```python
from build123d import *

# Parameters (mm, degrees)
SKETCH_1_R         = 7.5
EXTRUDE_1_DEPTH    = 4.5
SKETCH_9_R         = 2.25
EXTRUDE_6_DEPTH    = 1
EXTRUDE_2_DEPTH    = 5
SKETCH_6_R         = 1.75
EXTRUDE_3_DEPTH    = 0.5
SKETCH_7_R         = 1.5
EXTRUDE_4_DEPTH    = 5
SKETCH_8_R         = 8.5
SKETCH_8_R_2       = 7.5
EXTRUDE_5_DEPTH    = 1
HOLE_WIZARD_M3_1_D = 3.4


with BuildPart() as part:
    # ｽｹｯﾁ1 → ﾎﾞｽ - 押し出し1 (new body)
    with BuildSketch(Plane(origin=(0, 0, 0), x_dir=(1, 0, 0), z_dir=(0, 1, 0))):
        Circle(SKETCH_1_R)
    extrude(amount=EXTRUDE_1_DEPTH)

    # ｽｹｯﾁ9 → ﾎﾞｽ - 押し出し6 (add)
    with BuildSketch(Plane(origin=(0, 4.5, 0), x_dir=(1, 0, 0), z_dir=(0, 1, 0))):
        Circle(SKETCH_9_R)
    extrude(amount=EXTRUDE_6_DEPTH)

    # ｽｹｯﾁ2 → ﾎﾞｽ - 押し出し2 (add)
    with BuildSketch(Plane(origin=(0, 5.5, 0), x_dir=(1, 0, 0), z_dir=(0, 1, 0))):
        Polygon((2.020725942, 0), (1.010362971, 1.75), (-1.010362971, 1.75), (-2.020725942, 0), (-1.010362971, -1.75), (1.010362971, -1.75), align=None)
    extrude(amount=EXTRUDE_2_DEPTH)

    # ｽｹｯﾁ6 → ﾎﾞｽ - 押し出し3 (add)
    with BuildSketch(Plane(origin=(0, 10.5, 0), x_dir=(1, 0, 0), z_dir=(0, 1, 0))):
        Circle(SKETCH_6_R)
    extrude(amount=EXTRUDE_3_DEPTH)

    # ｽｹｯﾁ7 → ﾎﾞｽ - 押し出し4 (add)
    with BuildSketch(Plane(origin=(0, 11, 0), x_dir=(1, 0, 0), z_dir=(0, 1, 0))):
        Circle(SKETCH_7_R)
    extrude(amount=EXTRUDE_4_DEPTH)

    # ｽｹｯﾁ8 → ﾎﾞｽ - 押し出し5 (add)
    with BuildSketch(Plane(origin=(0, 0, 0), x_dir=(-1, 0, 0), z_dir=(0, -1, 0))):
        Circle(SKETCH_8_R)
        Circle(SKETCH_8_R_2, mode=Mode.SUBTRACT)
    extrude(amount=-EXTRUDE_5_DEPTH)

    # M3 すきま穴1 (through all)
    with Locations(Plane(origin=(0, 4.5, 0), x_dir=(1, 0, 0), z_dir=(0, 1, 0))):
        with Locations((0, 6), (0, -6)):
            Hole(HOLE_WIZARD_M3_1_D / 2)


solid = part.part
```
Verification items for the finished model (mm, model axes). A direction names the side the tool comes from. Give positions to 0.01 mm unless a question says otherwise; leave off trailing zeros. Write each loop counter-clockwise with the first axis right and the second up, starting at its lowest first coordinate (ties: lowest second). Pieces come first, ordered by that corner, then holes. Notation, with made-up numbers: (78.25, -15) - (99.25, -15) arc R7 cw to (99.25, -5) - close; hole circle Ø2 at (63.25, 47.25). An arc over 180 degrees is marked (long way). Put each result on its own line as item: value.
Q1. Section check B-B on y = 8.25. Record the cut outline in (x, z), and give its area (3 significant figures).
Result:
outline: (-2.02, 0) - (-1.01, -1.75) - (1.01, -1.75) - (2.02, 0) - (1.01, 1.75) - (-1.01, 1.75) - close
area: 10.6 mm2
Q2. Set-up check for faces 1 (the face through (-7.5, 2.73, -0.15)), 2 (the face through (-1.5, 13.46, -0.07)), 3 (the face through (-1.5, 8, -0.9)): record each of +Z, -Z, +X, -X, +Y, -Y from which the full face is reachable in a straight line by a thin tool's end or side.
Result:
face 1: -X, +Y
face 2: +Y
face 3: -Z, -X, +Y
Q3. Section check D-D on x = -3.75. Record the cut outline in (y, z), and give its area (3 significant figures).
Result:
outline: (0, -7.63) - (1, -7.63) - (1, -6.5) - (4.5, -6.5) - (4.5, 6.5) - (1, 6.5) - (1, 7.63) - (0, 7.63) - close
area: 60.7 mm2
Q4. Depth check by flat-ended pin: P1, Ø2, axis at x = 0.5, y = 9, coming from the +Z side; P2, Ø4, axis at y = 9.5, z = -3, coming from the +X side; P3, Ø4, axis at x = 1.5, y = 8, coming from the -Z side; P4, Ø2.5, axis at x = 0, z = 6, coming from the +Y side. Enter the tip coordinate at first touch or a pass-through.
Result:
P1: z = 1.75
P2: x = 1.44
P3: z = -1.75
P4: through
Q5. Section check A-A on z = 6.75. Record the cut outline in (x, y), and give its area (3 significant figures).
Result:
outline: (-5.17, 0) - (-1.53, 0) - (-1.53, 4.5) - (-3.27, 4.5) - (-3.27, 1) - (-5.17, 1) - close; (1.53, 0) - (5.17, 0) - (5.17, 1) - (3.27, 1) - (3.27, 4.5) - (1.53, 4.5) - close
area: 19.5 mm2
Q6. Scan lines: probe 1 along Y at (x, z) = (7.5, -2.5); probe 2 along Y at (x, z) = (4.5, -0.5); probe 3 along Z at (x, y) = (0, 1.7). Record each from-to range of solid material in increasing order. Write a range as from..to.
Result:
probe 1: 0..1
probe 2: 0..4.5
probe 3: -4.3..4.3
Q7. Section check C-C on x = 1.25. Count the separate pieces of the cut face and the enclosed holes in it, and give its area (3 significant figures).
Result:
separate pieces: 3
enclosed holes: 0
area: 74.4 mm2
Q8. Mould release check, pull along X, two halves, no side actions. Record for faces 4 (the face through (0.37, 2.22, -4.34)), 5 (the face through (0, 8, 1.75)), 6 (the face through (-4.57, 0.493, -7.167)): released by +X, released by -X, zero draft, split by the parting line, or undercut.
Result:
face 4: undercut
face 5: zero draft
face 6: split by the parting line
